Read the model definition and answer for the solid it produces. Units are mm, in the model's axes. Give positions to 0.01 mm unless a question says otherwise; leave off trailing zeros. Write each loop counter-clockwise with the first axis right and the second up, starting at its lowest first coordinate (ties: lowest second). Pieces come first, ordered by that corner, then holes. Notation, with made-up numbers: M -11.5,-31 L 29.5,-31 A34 cw 29.5,7 Z; hole C 84.5,54.5 d5. An arc over 180 degrees is marked long. Use a Markdown table: item, result. Add a question column.
Item 1: Consider probe 1 along Y at (x, z) = (0, 18); probe 2 along X at (y, z) = (-1, 27.5); probe 3 along Y at (x, z) = (-21.5, 17.5). Determine where each line is inside the solid, lowest interval first. Write a range as [from, to].
Item 2: The mould has two halves that part along X. Classify faces 1 (the flat face through (0, -7, 0)), 2 (the cylindrical face through (30.19, 9.51, 18.78)), 3 (the cylindrical face through (-0.619, -2.786, 18.783)): pulls with the +X half, pulls with the -X half, needs draft (parallel to the pull), parting line crosses it, or undercut.
Item 3: A cutting plane is placed at C-C on z = 17.5. Determine the outline of the cut face in (x, y), then the cut area to 3 significant figures.
Item 4: A cutting plane is placed at A-A on x = 0. Determine the outline of the cut face in (y, z).
Item 5: A cutting plane is placed at D-D on x = 21. Determine the outline of the cut face in (y, z).
Item 6: Given P1, Ø3, axis at y = -21.5, z = 6.5, coming from the +X side; P2, Ø12, axis at x = -1, z = 17, coming from the -Y side; P3, Ø5, axis at y = -20.5, z = 20, coming from the -X side, each flat-ended and moving along its own axis, determine where each tip first touches the part or whether it passes through.
from build123d import *

# Parameters (mm, degrees)
F0_R        = 31.6529983533
F0_R_2      = 16.2871330866
F0_R_3      = 2.853540911
F1_DEPTH    = 5.08
F2_DEPTH    = 25.4
F2_FACE_R   = 31.6529983533
F2_FACE_R_2 = 2.853540911
F3_DEPTH    = 7.62


with BuildPart() as f1:
    # F0 (on Top) → F1 (new body)
    with BuildSketch(Plane.XY):
        Circle(F0_R)
        Circle(F0_R_2, mode=Mode.SUBTRACT)
        Circle(F0_R_2)
        Circle(F0_R_3, mode=Mode.SUBTRACT)
    extrude(amount=F1_DEPTH)

    # F2 (add): a face of the model
    f2_faces = [f1.faces().sort_by_distance(p)[0] for p in [
        (-30.7577163621, 0, 5.08),
    ]]
    extrude(f2_faces, amount=F2_DEPTH)

    # F0 (on Top) + F2_face (on face) → F3 (join)
    with BuildSketch(Plane.XY):
        Circle(F0_R)
        Circle(F0_R_2, mode=Mode.SUBTRACT)
    with BuildSketch(Plane.XY.offset(30.48)):
        Circle(F2_FACE_R)
        Circle(F2_FACE_R_2, mode=Mode.SUBTRACT)
    extrude(amount=F3_DEPTH)


solid = f1.part
Filled in:
| question | item | result |
|---|---|---|
| 1 | probe 1 | [-31.65, -2.85], [2.85, 31.65] |
| 1 | probe 2 | [-31.64, -2.67], [2.67, 31.64] |
| 1 | probe 3 | [-23.23, 23.23] |
| 2 | face 1 | needs draft |
| 2 | face 2 | parting line crosses it |
| 2 | face 3 | undercut |
| 3 | outline | C 0,0 d63.31; hole C 0,0 d5.71 |
| 3 | area | 3,120 mm² |
| 4 | outline | M -31.65,0 L -2.85,0 L -2.85,38.1 L -31.65,38.1 Z; M 2.85,0 L 31.65,0 L 31.65,38.1 L 2.85,38.1 Z |
| 5 | outline | M -23.68,0 L 23.68,0 L 23.68,38.1 L -23.68,38.1 Z |
| 6 | P1 | x = 24.53 |
| 6 | P2 | y = -31.65 |
| 6 | P3 | x = -26.04 |
